Geometry: final body of the model. Coordinates: model frame, mm. Round coordinates to 2 decimals unless told otherwise and drop trailing zeros. Write each loop counter-clockwise with the first axis right and the second up, starting at its lowest first coordinate (ties: lowest second). Pieces come first, ordered by that corner, then holes. Notation, with made-up numbers: M -12,55 L -8,55 A17 cw -8,62 Z; hole C 30.5,-7 d10. An arc over 180 degrees is marked long. Use one line per item in the form item = value. Start each with the question number.
Item 1: Pin query (flat end, axial travel): pin 1 Ø5 at (y, z) = (1062.5, 7) entering from +X; pin 2 Ø5 at (y, z) = (814.5, 9) entering from -X; pin 3 Ø6 at (x, z) = (699, 9.5) entering from +Y. Return the tip coordinate at first contact, or that it passes through.
Item 2: Ray query, probe 1 along Y at (x, z) = (584, 6.5); probe 2 along X at (y, z) = (1043, 12.25); probe 3 along Y at (x, z) = (673, 8). Return the intervals inside material, ascending.
Item 3: Section query C-C (z = 4.25). State how many separate pieces and enclosed holes the cut face has, and give its area (3 significant figures).
Item 4: Section query B-B (y = 1033). Return loops of the section in (x, z).
Item 5: Section query D-D (x = 524.5). Return loops of the section in (y, z), and give its area (3 significant figures).
Item 6: Section query A-A (x = 590). Return loops of the section in (y, z), and give its area (3 significant figures).
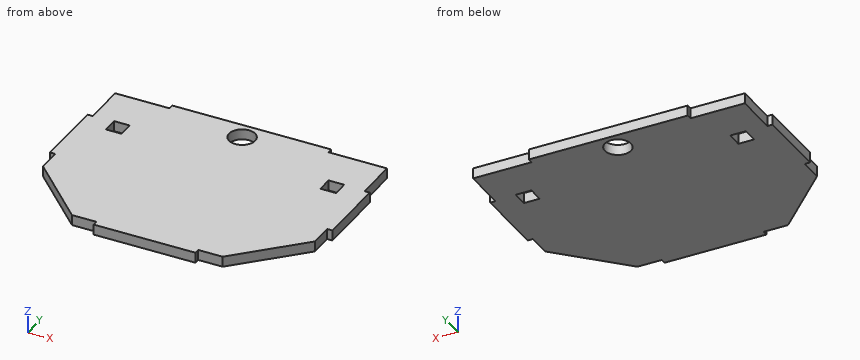
from build123d import *

# Parameters (mm, degrees)
BOSS_EXTRUDE1_DEPTH = 12.7
SKETCH2_R           = 15.875
SKETCH2_W           = 19.05
SKETCH2_H           = 19.05
CUT_EXTRUDE1_DEPTH  = 13.7


with BuildPart() as part:
    # Sketch1 → Boss-Extrude1 (new body)
    with BuildSketch(Plane.XY):
        Polygon((424.715446324, 892.207843626), (424.715446324, 920.715652439), (418.365446324, 920.715652439), (418.365446324, 1007.691853389), (424.715446324, 1007.691853389), (424.715446324, 1059.919118431), (490.806723979, 1059.919118431), (490.806723979, 1066.269118431), (683.70003755, 1066.269118431), (683.70003755, 1059.919118431), (754.915446324, 1059.919118431), (754.915446324, 1007.691853389), (761.265446324, 1007.691853389), (761.265446324, 920.715652439), (754.915446324, 920.715652439), (754.915446324, 892.207843626), (681.331146762, 818.667305174), (651.634447679, 818.667305174), (651.634447679, 812.317305174), (528.064815274, 812.317305174), (528.064815274, 818.667305174), (498.299745887, 818.667305174), align=None)
    extrude(amount=BOSS_EXTRUDE1_DEPTH)

    # Sketch2 → Cut-Extrude1 (cut, through all)
    with BuildSketch(Plane.XY.offset(12.7)):
        with Locations((587.253380764, 1044.044118431)):
            Circle(SKETCH2_R)
        with Locations((459.640446324, 999.594118431)):
            Rectangle(SKETCH2_W, SKETCH2_H)
        with Locations((719.990446324, 999.594118431)):
            Rectangle(SKETCH2_W, SKETCH2_H)
    extrude(amount=-CUT_EXTRUDE1_DEPTH, mode=Mode.SUBTRACT)


solid = part.part
Working result:
q1.pin_1 = 683.7
q1.pin_2 = 528.06
q1.pin_3 = 1059.92
q2.probe_1 = 812.32 to 1028.51, 1059.58 to 1066.27
q2.probe_2 = 424.72 to 571.41, 603.09 to 754.92
q2.probe_3 = 818.67 to 1066.27
q3.separate_pieces = 1
q3.enclosed_holes = 3
q3.area = 75,800 mm²
q4.outline = M 424.72,0 L 575.85,0 L 575.85,12.7 L 424.72,12.7 Z; M 598.66,0 L 754.92,0 L 754.92,12.7 L 598.66,12.7 Z
q5.outline = M 818.67,0 L 1066.27,0 L 1066.27,12.7 L 818.67,12.7 Z
q5.area = 3,140 mm²
q6.outline = M 812.32,0 L 1028.41,0 L 1028.41,12.7 L 812.32,12.7 Z; M 1059.68,0 L 1066.27,0 L 1066.27,12.7 L 1059.68,12.7 Z
q6.area = 2,830 mm²
